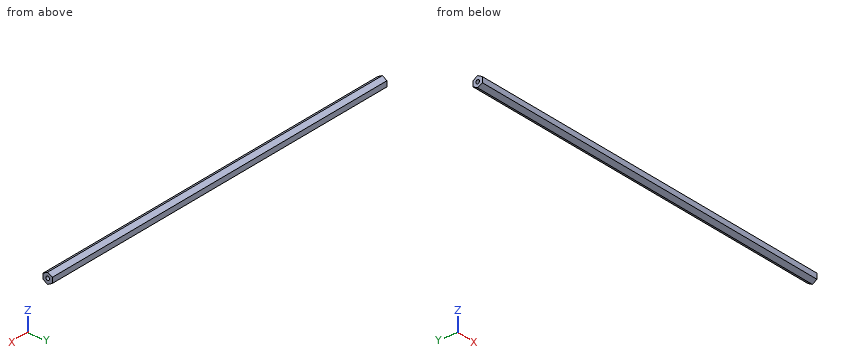
```python
from build123d import *

# Parameters (mm, degrees)
BOSS_EXTRUDE1_DEPTH         = 525.4625
F_1_4_20_TAPPED_HOLE1_D     = 5.1054
F_1_4_20_TAPPED_HOLE1_DEPTH = 16.51
F_1_4_20_TAPPED_HOLE1_TIP   = 1.533816902
F_1_4_20_TAPPED_HOLE2_D     = 5.1054
F_1_4_20_TAPPED_HOLE2_DEPTH = 16.51
F_1_4_20_TAPPED_HOLE2_TIP   = 1.533816902


with BuildPart() as part:
    # Sketch1 → Boss-Extrude1 (new body)
    with BuildSketch(Plane(origin=(0, 0, 0), x_dir=(0, 0, -1), z_dir=(1, 0, 0))):
        Polygon((7.332348419, 0), (3.666174209, 6.35), (-3.666174209, 6.35), (-7.332348419, 0), (-3.666174209, -6.35), (3.666174209, -6.35), align=None)
    extrude(amount=BOSS_EXTRUDE1_DEPTH)

    # 1/4-20 Tapped Hole1
    with Locations(Plane(origin=(525.4625, 0, 0), x_dir=(0, 0, -1), z_dir=(1, 0, 0))):
        with Locations((0, 0)):
            Hole(F_1_4_20_TAPPED_HOLE1_D / 2, depth=F_1_4_20_TAPPED_HOLE1_DEPTH)
            with Locations((0, 0, -(F_1_4_20_TAPPED_HOLE1_DEPTH + F_1_4_20_TAPPED_HOLE1_TIP / 2))):  # 118° drill point
                Cone(0, F_1_4_20_TAPPED_HOLE1_D / 2, F_1_4_20_TAPPED_HOLE1_TIP, mode=Mode.SUBTRACT)

    # 1/4-20 Tapped Hole2
    with Locations(Plane.ZY):
        with Locations((0, 0)):
            Hole(F_1_4_20_TAPPED_HOLE2_D / 2, depth=F_1_4_20_TAPPED_HOLE2_DEPTH)
            with Locations((0, 0, -(F_1_4_20_TAPPED_HOLE2_DEPTH + F_1_4_20_TAPPED_HOLE2_TIP / 2))):  # 118° drill point
                Cone(0, F_1_4_20_TAPPED_HOLE2_D / 2, F_1_4_20_TAPPED_HOLE2_TIP, mode=Mode.SUBTRACT)


solid = part.part
```
CAD build for the part. Positions are in the model's coordinates, mm. Round coordinates to 2 decimals unless told otherwise and drop trailing zeros. Loops run counter-clockwise (first coordinate to the right, second up) from the corner with the lowest first, then second, coordinate; pieces in that order, holes last. Notation, with made-up numbers: (22.25, 9) - (73.25, 9) arc R11 ccw to (73.25, 20) - close; hole circle Ø5 at (31.25, -7.75). An arc over 180 degrees is marked (long way). Return JSON: item names as keys, results as strings. Group by question number.
Q1. Drill centre lines: line 1 along Y through (x, z) = (7.5, 0); line 2 along Z through (x, y) = (518.5, 0); line 3 along Z through (x, y) = (273, 3.5). Where is each one in solid material? Low to high. Write a range as [from, to].
Q2. Flat gauge pins, fed straight in: pin 1 Ø1 at (x, y) = (203.5, -4.5) entering from +Z; pin 2 Ø2 at (x, y) = (106.5, 3.5) entering from +Z; pin 3 Ø5 at (x, y) = (332.5, -2) entering from +Z. Where does each tip first touch, or does it go through?
Q3. Band-saw the part on A-A on x = 223. Give the cut face in (y, z), plus the area to 3 significant figures.
Solutions:
{
 "1": {"line 1": "y = [-6.35, -2.55], [2.55, 6.35]", "line 2": "z = [-7.33, -2.55], [2.55, 7.33]", "line 3": "z = [-5.31, 5.31]"},
 "2": {"pin 1": "stops at z = 5.02", "pin 2": "stops at z = 5.89", "pin 3": "stops at z = 7.33"},
 "3": {"outline": "(-6.35, -3.67) - (0, -7.33) - (6.35, -3.67) - (6.35, 3.67) - (0, 7.33) - (-6.35, 3.67) - close", "area": "140 mm^2"}
}
